The model under review builds one solid part; all positions refer to its coordinate system, in mm. Coordinates: 2 decimals unless noted, no trailing zeros. Write each loop counter-clockwise with the first axis right and the second up, starting at its lowest first coordinate (ties: lowest second). Pieces come first, ordered by that corner, then holes. Notation, with made-up numbers: (-39.75, 8.5) - (2.25, 8.5) arc R20 ccw to (2.25, 24.5) - close; hole circle Ø7 at (-28, 34). An arc over 180 degrees is marked (long way). Return JSON: item names as keys, results as strings. Group by question number.
(1) To check wall thickness, follow L1, parallel to Z at x = 13, y = 29; L2, parallel to X at y = 3, z = 133.5; L3, parallel to Y at x = 8.5, z = 31. State the ranges of each line that lie inside material, in increasing order. Write a range as from..to.
(2) We need section C-C on x = 37.5. State the section outline as (y, z) points, then the cut area to 3 significant figures.
(3) We need section D-D on x = -36. State the section outline as (y, z) points, then the cut area to 3 significant figures.
(4) We need section A-A on x = 0. State the section outline as (y, z) points, then the cut area to 3 significant figures.
(5) For pin 1 Ø5 at (x, y) = (-22.5, -9) entering from +Z; pin 2 Ø5 at (x, z) = (-33.5, -111.5) entering from +Y; pin 3 Ø3 at (x, z) = (-33, -286) entering from +Y; pin 4 Ø4 at (x, z) = (10.5, -373.5) entering from +Y, all flat-tipped, find the tip position at first contact; note any pin that passes through.
```python
from build123d import *

# Parameters (mm, degrees)
SKETCH1_R           = 50.8
BOSS_EXTRUDE1_DEPTH = 350
SKETCH2_R           = 8
BOSS_EXTRUDE2_DEPTH = 370
SKETCH3_R           = 8
BOSS_EXTRUDE3_DEPTH = 95


with BuildPart() as part:
    # Sketch1 → Boss-Extrude1 (new, symmetric)
    with BuildSketch(Plane.XY):
        Circle(SKETCH1_R)
    extrude(amount=BOSS_EXTRUDE1_DEPTH, both=True)

    # Sketch2 → Boss-Extrude2 (add, symmetric)
    with BuildSketch(Plane.XY):
        Circle(SKETCH2_R)
    extrude(amount=BOSS_EXTRUDE2_DEPTH, both=True)

    # Sketch3 → Boss-Extrude3 (add)
    with BuildSketch(Plane(origin=(0, 0, -370), x_dir=(-1, 0, 0), z_dir=(0, 0, -1))):
        Circle(SKETCH3_R)
    extrude(amount=BOSS_EXTRUDE3_DEPTH)


solid = part.part
```
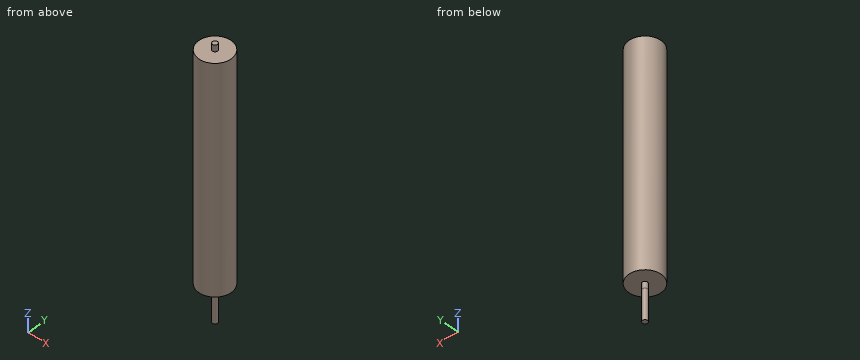
Ans:
{
 "1": {"L1": "-350..350", "L2": "-50.71..50.71", "L3": "-50.08..50.08"},
 "2": {"outline": "(-34.27, -350) - (34.27, -350) - (34.27, 350) - (-34.27, 350) - close", "area": "48,000 mm²"},
 "3": {"outline": "(-35.84, -350) - (35.84, -350) - (35.84, 350) - (-35.84, 350) - close", "area": "50,200 mm²"},
 "4": {"outline": "(-50.8, -350) - (-8, -350) - (-8, -465) - (8, -465) - (8, -350) - (50.8, -350) - (50.8, 350) - (8, 350) - (8, 370) - (-8, 370) - (-8, 350) - (-50.8, 350) - close", "area": "73,300 mm²"},
 "5": {"pin 1": "z = 350", "pin 2": "y = 40.24", "pin 3": "y = 39.85", "pin 4": "through"}
}
